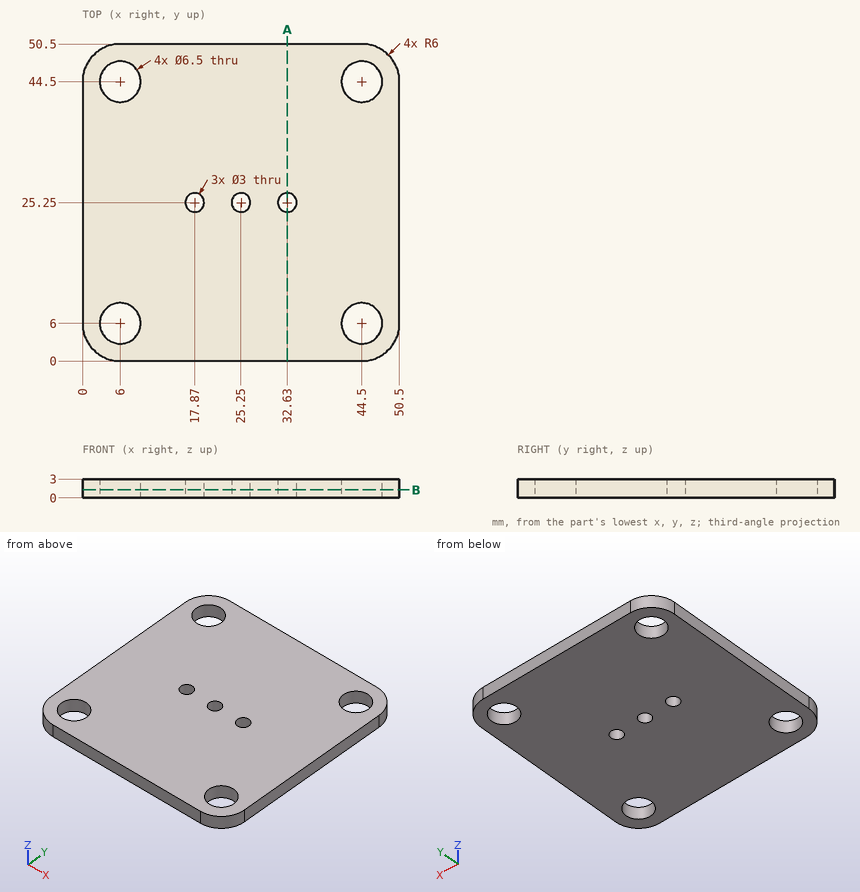
Could you check a few things on this drawing? It's one solid part, dimensions in mm from its lowest x, y, z. Coordinates: 2 decimals unless noted, no trailing zeros. Order: outer loops, then holes, each group sorted by start corner. A loop starts at its lowest first (then second) coordinate and runs counter-clockwise, first axis right, second up.
1) I need wall thicknesses on line 1 (Y direction, x = 32.63, z = 0.6); line 2 (Y direction, x = 41.5, z = 2.45); line 3 (Y direction, x = 43, z = 2.85). Which ranges of each line are inside material? Lowest first, please.
2) Imagine slicing it at A-A on x = 32.63. List the corners of the cut face in (y, z) for me.
3) Imagine slicing it at B-B on z = 1.25. List the corners of the cut face in (x, y) for me.
4) Will this pin go through, and if not, where does the flat tip stop? pin 1 (3.5 mm diameter, centred on x = 32.63, y = 25.25, fed in from -Z).
Response values:
1. line 1: y = 0 to 23.75, 26.75 to 50.5
1. line 2: y = 0 to 4.75, 7.25 to 43.25, 45.75 to 50.5
1. line 3: y = 0 to 3.12, 8.88 to 41.62, 47.38 to 50.5
2. outline: (0, 0) - (23.75, 0) - (23.75, 3) - (0, 3) - close; (26.75, 0) - (50.5, 0) - (50.5, 3) - (26.75, 3) - close
3. outline: (0, 6) arc R6 ccw to (6, 0) - (44.5, 0) arc R6 ccw to (50.5, 6) - (50.5, 44.5) arc R6 ccw to (44.5, 50.5) - (6, 50.5) arc R6 ccw to (0, 44.5) - close; hole circle Ø6.5 at (6, 6); hole circle Ø6.5 at (6, 44.5); hole circle Ø3 at (17.87, 25.25); hole circle Ø3 at (25.25, 25.25); hole circle Ø3 at (32.63, 25.25); hole circle Ø6.5 at (44.5, 6); hole circle Ø6.5 at (44.5, 44.5)
4. pin 1: stops at z = 0
